Can you work these out from the drawing? Everything is in mm from the part's minimum corner. A direction names the side the tool comes from. Coordinates: 2 decimals unless noted, no trailing zeros. Order: outer loops, then holes, each group sorted by start corner. A loop starts at its lowest first (then second) coordinate and runs counter-clockwise, first axis right, second up. Notation, with made-up numbers: M 73.5,76 L 117.5,76 A20 cw 117.5,112 Z; hole C 78,75.5 d8. An arc over 180 degrees is marked long. One line per question, with ' | ' between items. Start each with the question number.
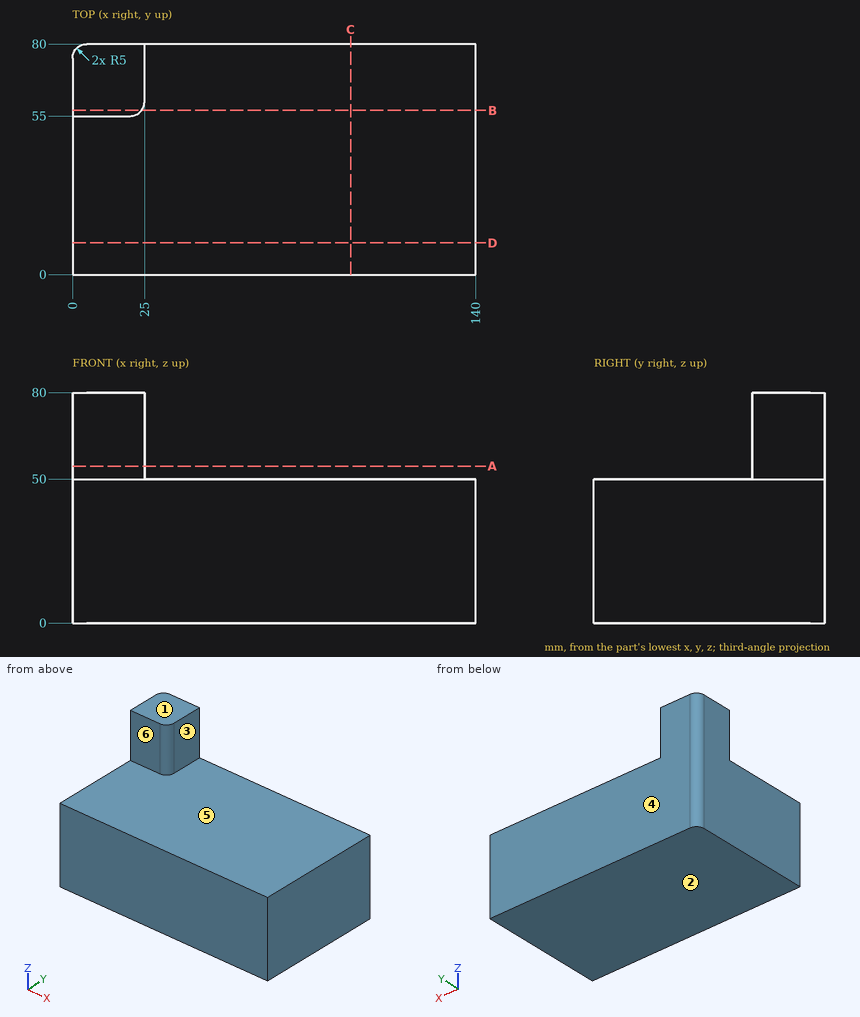
(1) If I drill on line 1 along Z through (x, y) = (119.5, 35); line 2 along X through (y, z) = (65.5, 56.5); line 3 along X through (y, z) = (76, 37), over which ranges is the centre line in solid material (lowest first)? Write a range as from..to.
(2) On a 3-axis mill with a long thin cutter (end or side, diameter ignored), from which of +Z, -Z, +X, -X, +Y, -Y can I reach the whole of each face in a straight line? I mean the marked faces 4, 5 and 6. Say none if no direction works.
(3) Imagine slicing it at C-C, the plane x = 96.5. Write out the boundary of the cut face in (y, z), plus the area to 3 significant figures.
(4) Imagine slicing it at B-B, the plane y = 57. Write out the boundary of the cut face in (x, z).
(5) For P1, Ø12, axis at x = 122.5, y = 35.5, coming from the +Z side; P2, Ø10, axis at x = 13, z = 70.5, coming from the -Y side; P3, Ø6, axis at y = 69, z = 63, coming from the +X side, each with a flat end and sliding along its axis, tell me the tip position at first contact or that it passes through.
(6) Imagine slicing it at D-D, the plane y = 11. Write out the boundary of the cut face in (x, z).
(7) We'd pull the mould along Z, two halves only. Please class the marked faces 1, 2 and 3: +Z half, -Z half, draft (parallel to the pull), parting line (faces both ways), or undercut.
(8) Imagine slicing it at A-A, the plane z = 54.5. Write out the boundary of the cut face in (x, y).
Answers:
1) line 1: 0..50 | line 2: 0..25 | line 3: 0.1..140
2) face 4: +Z, -Z, +X, -X, +Y | face 5: +Z, +X, -Y | face 6: +Z, +X, -X, -Y
3) outline: M 0,0 L 80,0 L 80,50 L 0,50 Z | area: 4,000 mm²
4) outline: M 0,0 L 140,0 L 140,50 L 24,50 L 24,80 L 0,80 Z
5) P1: z = 50 | P2: y = 55 | P3: x = 25
6) outline: M 0,0 L 140,0 L 140,50 L 0,50 Z
7) face 1: +Z half | face 2: -Z half | face 3: draft
8) outline: M 0,55 L 20,55 A5 ccw 25,60 L 25,80 L 5,80 A5 ccw 0,75 Z
